Work out the finished part from the listing and answer in its coordinate system (mm). Coordinates: 2 decimals unless noted, no trailing zeros. Loops run counter-clockwise (first coordinate to the right, second up) from the corner with the lowest first, then second, coordinate; pieces in that order, holes last. Notation, with made-up numbers: (0.5, -28) - (21.5, -28) arc R36 ccw to (21.5, 10) - close; hole circle Ø7 at (57, -32). An arc over 180 degrees is marked (long way). Write each question's results on one line, items separated by ' | '. Start each with the question number.
1. Find the intervals of material crossed by line 1 along Z through (x, y) = (-2.75, 91); line 2 along X through (y, z) = (185, 4.45) (3 decimals), in increasing order. Write a range as [from, to].
2. A cutting plane is placed at D-D on x = 0. State how many separate pieces and enclosed holes the cut face has, then the cut area to 3 significant figures.
3. This flat-tipped pin is pushed along its axis until it touches: P1, Ø3.5, axis at x = 0, y = 20, coming from the -Z side. Where does it stop, or does it pass through?
4. A cutting plane is placed at B-B on z = -1.5. Determine the outline of the cut face in (x, y), then the cut area to 3 significant figures.
5. A cutting plane is placed at C-C on y = 100. Determine the outline of the cut face in (x, z), then the cut area to 3 significant figures.
6. A cutting plane is placed at A-A on y = 120. Determine the outline of the cut face in (x, z) (3 decimals).
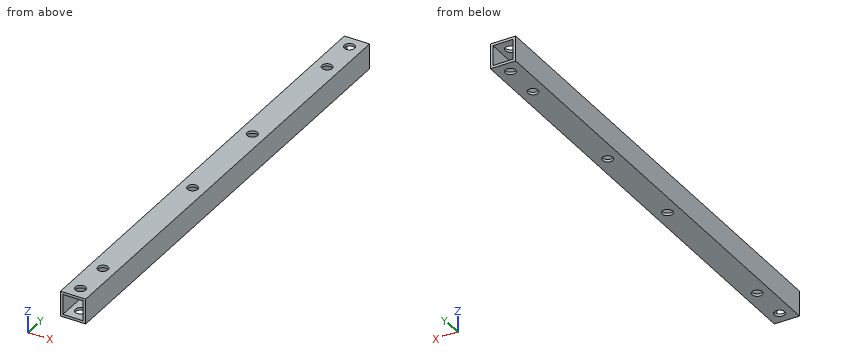
from build123d import *

# Parameters (mm, degrees)
SKETCH1_W           = 10
SKETCH1_H           = 10
SKETCH1_W_2         = 8
SKETCH1_H_2         = 8
BOSS_EXTRUDE1_DEPTH = 190
SKETCH2_R           = 2.025
CUT_EXTRUDE1_DEPTH  = 191.328663107
SKETCH3_R           = 2.025
CUT_EXTRUDE2_DEPTH  = 191.328663107


with BuildPart() as part:
    # Sketch1 → Boss-Extrude1 (new body)
    with BuildSketch(Plane(origin=(0, 0, 0), x_dir=(1, 0, 0), z_dir=(0, 1, 0))):
        Rectangle(SKETCH1_W, SKETCH1_H)
        Rectangle(SKETCH1_W_2, SKETCH1_H_2, mode=Mode.SUBTRACT)
    extrude(amount=BOSS_EXTRUDE1_DEPTH)

    # Sketch2 → Cut-Extrude1 (cut, through all)
    with BuildSketch(Plane.XY.offset(5)):
        with Locations((0, 120)):
            Circle(SKETCH2_R)
        with Locations((0, 80)):
            Circle(SKETCH2_R)
    extrude(amount=-CUT_EXTRUDE1_DEPTH, mode=Mode.SUBTRACT)

    # Sketch3 → Cut-Extrude2 (cut, through all)
    with BuildSketch(Plane.XY.offset(5)):
        with Locations((0, 185)):
            Circle(SKETCH3_R)
        with Locations((0, 170)):
            Circle(SKETCH3_R)
        with Locations((0, 5)):
            Circle(SKETCH3_R)
        with Locations((0, 20)):
            Circle(SKETCH3_R)
    extrude(amount=-CUT_EXTRUDE2_DEPTH, mode=Mode.SUBTRACT)


solid = part.part
Values:
1) line 1: [-5, -4], [4, 5] | line 2: [-5, -2.025], [2.025, 5]
2) separate pieces: 14 | enclosed holes: 0 | area: 331 mm^2
3) P1: through
4) outline: (-5, 0) - (-4, 0) - (-4, 190) - (-5, 190) - close; (4, 0) - (5, 0) - (5, 190) - (4, 190) - close | area: 380 mm^2
5) outline: (-5, -5) - (5, -5) - (5, 5) - (-5, 5) - close; hole (-4, -4) - (4, -4) - (4, 4) - (-4, 4) - close | area: 36.0 mm^2
6) outline: (-5, -5) - (-2.025, -5) - (-2.025, -4) - (-4, -4) - (-4, 4) - (-2.025, 4) - (-2.025, 5) - (-5, 5) - close; (2.025, -5) - (5, -5) - (5, 5) - (2.025, 5) - (2.025, 4) - (4, 4) - (4, -4) - (2.025, -4) - close
